from build123d import *

# Parameters (mm, degrees)
CROQUIS1_W              = 76.2
CROQUIS1_H              = 1000
SALIENTE_EXTRUIR1_DEPTH = 76.2
CROQUIS2_W              = 136.2
CROQUIS2_H              = 136.2
SALIENTE_EXTRUIR2_DEPTH = 9.525
CROQUIS3_W              = 526.2
CROQUIS3_H              = 420
SALIENTE_EXTRUIR3_DEPTH = 200
CROQUIS4_R              = 19.05
SALIENTE_EXTRUIR4_DEPTH = 30
CROQUIS5_R              = 19.05


with BuildPart() as part:
    # Croquis1 → Saliente-Extruir1 (new body)
    with BuildSketch(Plane.XY):
        with Locations((38.1, 500)):
            Rectangle(CROQUIS1_W, CROQUIS1_H)
    extrude(amount=SALIENTE_EXTRUIR1_DEPTH)

    # Croquis2 → Saliente-Extruir2 (add)
    with BuildSketch(Plane.XZ):
        with Locations((38.1, 38.1)):
            Rectangle(CROQUIS2_W, CROQUIS2_H)
    extrude(amount=-SALIENTE_EXTRUIR2_DEPTH)

    # Croquis3 → Saliente-Extruir3 (add)
    with BuildSketch(Plane.XY.offset(76.2)):
        with Locations((63.1, 790)):
            Rectangle(CROQUIS3_W, CROQUIS3_H)
    extrude(amount=SALIENTE_EXTRUIR3_DEPTH)

    # Croquis4 → Saliente-Extruir4 (add)
    with BuildSketch(Plane.XZ.offset(-580)):
        with Locations(Location((261.2, 176.2, 0), (0, 0, 90))):
            Circle(CROQUIS4_R)
    extrude(amount=SALIENTE_EXTRUIR4_DEPTH)

    # Barrer1: sweep along a curve in space
    with BuildLine() as barrer1_path:
        Line((261.2, 550, 176.2), (261.2, 280, 176.2))
        ThreePointArc((261.2, 280, 176.2), (261.2, 258.786796564, 167.413203436), (261.2, 250, 146.2))
        Line((261.2, 250, 146.2), (261.2, 250, 56.2))
        ThreePointArc((261.2, 250, 56.2), (269.986796564, 250, 34.986796564), (291.2, 250, 26.2))
        Line((291.2, 250, 26.2), (531.2, 250, 26.2))
        ThreePointArc((531.2, 250, 26.2), (552.413203436, 250, 34.986796564), (561.2, 250, 56.2))
        Line((561.2, 250, 56.2), (561.2, 250, 96.2))
        ThreePointArc((561.2, 250, 96.2), (561.2, 258.786796564, 117.413203436), (561.2, 280, 126.2))
        Line((561.2, 280, 126.2), (561.2, 520, 126.2))
        ThreePointArc((561.2, 520, 126.2), (561.2, 541.213203436, 134.986796564), (561.2, 550, 156.2))
        Line((561.2, 550, 156.2), (561.2, 550, 476.2))
    # Croquis5 → Barrer1 (sweep)
    with BuildSketch(Plane.XZ.offset(-550)):
        with Locations((261.2, 176.2)):
            Circle(CROQUIS5_R)
    sweep(path=barrer1_path.line)


solid = part.part
The model under review builds one solid part; all positions refer to its coordinate system, in mm. A direction names the side the tool comes from. Give positions to 0.01 mm unless a question says otherwise; leave off trailing zeros. Write each loop counter-clockwise with the first axis right and the second up, starting at its lowest first coordinate (ties: lowest second). Pieces come first, ordered by that corner, then holes.
1. Wall thickness on L1, parallel to Y at x = 263.5, z = 102; L2, parallel to Z at x = 264.5, y = 851.5; L3, parallel to X at y = 808.5, z = 202.5: over which ranges is each line inside the solid? List them lowest first.
2. Tool access review of faces 5 (the flat face through (326.2, 787, 175)), 6 (the flat face through (38, 512, 0)), 7 (the cylindrical face through (278.88, 427.9, 183.29)): name each direction out of +Z, -Z, +X, -X, +Y, -Y from which nothing blocks a thin tool from reaching the whole face with its end or side.
3. Draft analysis for pull direction X (two halves, no side actions). For faces 1 (the flat face through (199, 793, 76.2)), 2 (the cylindrical face through (247.159, 237.125, 100.57)), 3 (the flat face through (0, 498, 38)), 4 (the cylindrical face through (412.88, 231.112, 23.72)), state which applies: +X half, -X half, draft (parallel to the pull), parting line (faces both ways), or undercut.
4. Add section C-C, the plane y = 493. Count the separate pieces of the cut face and the enclosed holes in it, plus the area to 3 significant figures.
5. For P1, Ø10.5, axis at x = 39, y = 3, coming from the +Z side; P2, Ø10.5, axis at y = 3, z = 8.5, coming from the +X side; P3, Ø8, axis at x = 147.5, z = 262, coming from the -Y side, all flat-tipped, find the tip position at first contact; note any pin that passes through.
6. Add section A-A, the plane x = 25. Write out the cut boundary in (y, z) (3 decimals).
7. Add section B-B, the plane y = 711.5. Write out the cut boundary in (x, z), plus the area to 3 significant figures.
8. Add section D-D, the plane x = 505.5. Write out the cut boundary in (y, z), plus the area to 3 significant figures.
Worked answers:
1. L1: y = 231.09 to 268.91, 580 to 1000
1. L2: z = 76.2 to 276.2
1. L3: x = -200 to 326.2
2. face 5: +Z, -Z, +X, +Y, -Y
2. face 6: -Z, +X, -X, +Y
2. face 7: none
3. face 1: draft
3. face 2: undercut
3. face 3: -X half
3. face 4: undercut
4. separate pieces: 3
4. enclosed holes: 0
4. area: 8,090 mm2
5. P1: stops at z = 106.2
5. P2: stops at x = 106.2
5. P3: stops at y = 580
6. outline: (0, -30) - (9.525, -30) - (9.525, 0) - (1000, 0) - (1000, 276.2) - (580, 276.2) - (580, 76.2) - (9.525, 76.2) - (9.525, 106.2) - (0, 106.2) - close
7. outline: (-200, 76.2) - (0, 76.2) - (0, 0) - (76.2, 0) - (76.2, 76.2) - (326.2, 76.2) - (326.2, 276.2) - (-200, 276.2) - close
7. area: 111,000 mm2
8. outline: circle Ø38.1 at (250, 26.2)
8. area: 1,140 mm2
